Input: part model. Units: mm. Frame: model coordinates. Face numbers are marked on the shaded views. A direction names the side the tool comes from. Coordinates: 2 decimals unless noted, no trailing zeros. Write each loop counter-clockwise with the first axis right and the second up, starting at its lowest first coordinate (ties: lowest second). Pieces come first, ordered by that corner, then holes. Notation, with made-up numbers: (60.25, -33) - (102.25, -33) arc R7 cw to (102.25, -25) - close; hole circle Ø6 at (-4.75, 72.25). An arc over 180 degrees is marked (long way). Use a Markdown table: item, result. Add a question column.
Q1. Section query C-C (z = 7.75). Return the cut outline in (x, y), then the cut area to 3 significant figures.
Q2. Pin query (flat end, axial travel): P1, Ø3, axis at x = 1, z = 4, coming from the +Y side; P2, Ø3.5, axis at y = 19, z = 1, coming from the -X side; P3, Ø3.5, axis at x = -14.5, z = 1.5, coming from the -Y side. Return the tip coordinate at first contact, or that it passes through.
Q3. Set-up query: the marked faces 1, 2, 3, 4 and 5. Return all of +Z, -Z, +X, -X, +Y, -Y with unobstructed straight access to the full face (end or side cutting, diameter ignored); none if empty.
Q4. Material intervals for probe 1 along Y at (x, z) = (0, 4.5); probe 2 along Y at (x, z) = (-0.5, 2.75); probe 3 along Z at (x, y) = (-8.5, -0.5), sorted ascending. Write a range as from..to.
Q5. Section query A-A (x = 0). Return the cut outline in (y, z), then the cut area to 3 significant figures.
Q6. Mould query, pull axis X, two halves, no side actions, for the marked faces 6, 7 and 8. Classes: released by +X, released by -X, zero draft, split by the parting line, or undercut.
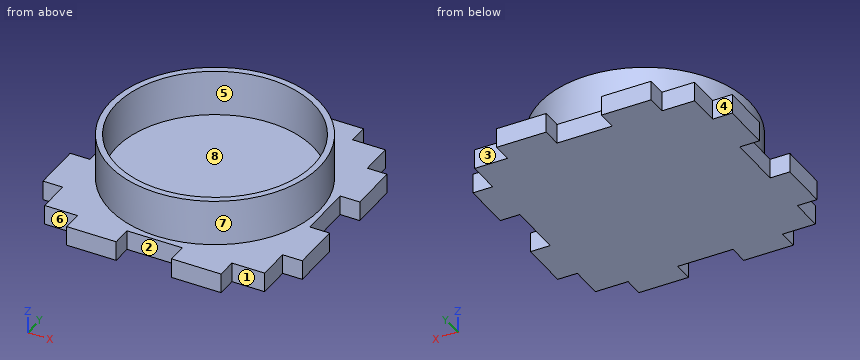
from build123d import *

# Parameters (mm, degrees)
F0_W     = 34
F0_H     = 34
F1_DEPTH = 3
F2_W     = 3
F2_H     = 8
F2_W_2   = 8
F2_H_2   = 3
F3_DEPTH = 3
F4_W     = 51.87688
F4_H     = 52.158144
F5_DEPTH = 3.001
F6_R     = 16
F6_R_2   = 15.05
F7_DEPTH = 7


with BuildPart() as f1:
    # F0 (on Top) → F1 (new body)
    with BuildSketch(Plane.XY):
        Rectangle(F0_W, F0_H)
    extrude(amount=F1_DEPTH)

    # F2 (on face) → F3 (join)
    with BuildSketch(Plane.XY.offset(3)):
        with Locations((-18.5, 8)):
            Rectangle(F2_W, F2_H)
        with Locations((-18.5, -8)):
            Rectangle(F2_W, F2_H)
        with Locations((-8, -18.5)):
            Rectangle(F2_W_2, F2_H_2)
        with Locations((8, -18.5)):
            Rectangle(F2_W_2, F2_H_2)
        with Locations((18.5, -8)):
            Rectangle(F2_W, F2_H)
        with Locations((18.5, 8)):
            Rectangle(F2_W, F2_H)
        with Locations((8, 18.5)):
            Rectangle(F2_W_2, F2_H_2)
        with Locations((-8, 18.5)):
            Rectangle(F2_W_2, F2_H_2)
    extrude(amount=-F3_DEPTH)

    # F4 (on face) → F5 (cut, through all)
    with BuildSketch(Plane.XY.offset(3)):
        Rectangle(F4_W, F4_H)
        Polygon((16.78, -16.78), (11.78, -16.78), (11.78, -19.78), (4.22, -19.78), (4.22, -16.78), (-4.22, -16.78), (-4.22, -19.78), (-11.78, -19.78), (-11.78, -16.78), (-16.78, -16.78), (-16.78, -11.78), (-19.78, -11.78), (-19.78, -4.22), (-16.78, -4.22), (-16.78, 4.22), (-19.78, 4.22), (-19.78, 11.78), (-16.78, 11.78), (-16.78, 16.78), (-11.78, 16.78), (-11.78, 19.78), (-4.22, 19.78), (-4.22, 16.78), (4.22, 16.78), (4.22, 19.78), (11.78, 19.78), (11.78, 16.78), (16.78, 16.78), (16.78, 11.78), (19.78, 11.78), (19.78, 4.22), (16.78, 4.22), (16.78, -4.22), (19.78, -4.22), (19.78, -11.78), (16.78, -11.78), align=None, mode=Mode.SUBTRACT)
    extrude(amount=-F5_DEPTH, mode=Mode.SUBTRACT)

    # F6 (on face) → F7 (join)
    with BuildSketch(Plane.XY.offset(3)):
        Circle(F6_R)
        Circle(F6_R_2, mode=Mode.SUBTRACT)
    extrude(amount=F7_DEPTH)


solid = f1.part
Values follow:
| question | item | result |
|---|---|---|
| 1 | outline | circle Ø32 at (0, 0); hole circle Ø30.1 at (0, 0) |
| 1 | area | 92.7 mm2 |
| 2 | P1 | y = 16.78 |
| 2 | P2 | x = -11.78 |
| 2 | P3 | y = -16.78 |
| 3 | face 1 | +Z, -Z, +X, -Y |
| 3 | face 2 | +Z, -Z, -Y |
| 3 | face 3 | +Z, -Z, +X, +Y |
| 3 | face 4 | +Z, -Z, -X, +Y |
| 3 | face 5 | +Z |
| 4 | probe 1 | -16..-15.05, 15.05..16 |
| 4 | probe 2 | -16.78..16.78 |
| 4 | probe 3 | 0..3 |
| 5 | outline | (-16.78, 0) - (16.78, 0) - (16.78, 3) - (16, 3) - (16, 10) - (15.05, 10) - (15.05, 3) - (-15.05, 3) - (-15.05, 10) - (-16, 10) - (-16, 3) - (-16.78, 3) - close |
| 5 | area | 114 mm2 |
| 6 | face 6 | zero draft |
| 6 | face 7 | split by the parting line |
| 6 | face 8 | undercut |
